Build history of the part. All positions in model axes, mm. A direction names the side the tool comes from. Round coordinates to 2 decimals unless told otherwise and drop trailing zeros. Order: outer loops, then holes, each group sorted by start corner. A loop starts at its lowest first (then second) coordinate and runs counter-clockwise, first axis right, second up. Notation, with made-up numbers: (-25, -26) -> (-9, -26) arc R8 ccw to (-9, -15) -> close; hole circle Ø4 at (73.5, 5). An arc over 180 degrees is marked (long way). Write item = value, one per line.
Autodesk Inventor part; units mm, degrees
ref_plane "Начальная плоскость" through (0, 0, -16.5685) normal (0, 0, 1) x (1, 0, 0)
ref_plane "Конечная плоскость" through (0, 0, 346.57) normal (0, 0, 1) x (1, 0, 0)
ref_plane "РабПлоскость4" through (21.07, -40, 346.57) normal (0, 0.7071, 0.7071) x (1, 0, 0)
ref_plane "Начальная плоскость" through (0, 0, -16.5685) normal (0, 0, 1) x (1, 0, 0)
ref_plane "Конечная плоскость" through (0, 0, 346.57) normal (0, 0, 1) x (1, 0, 0)
sketch "Эскиз" plane through (0, 0, 0) normal (0, 0, 1) x (1, 0, 0)
  line L0 (-1.43, 0) -> (-1.43, 40)
  line L1 (-1.43, 40) -> (43.57, 40)
  line L2 (43.57, 40) -> (43.57, 38.1774)
  line L3 (39.9881, 34.1993) -> (11.2338, 31.1771)
  line L4 (4.07, 23.221) -> (4.07, 0)
  line L5 (4.07, 0) -> (-1.43, 0) construction
  line L6 (23.82, 40) -> (23.82, 32.5) construction
  line L7 (43.57, 34.5758) -> (43.57, 32.5) construction
  line L8 (43.57, 32.5) -> (23.82, 32.5) construction
  line L9 (0, 15) -> (0, -27) construction
  line L10 (-5.539, 0) -> (16.0067, 0) construction
  line L11 (-1.43, 0) -> (-1.43, -40)
  line L12 (-1.43, -40) -> (43.57, -40)
  line L13 (43.57, -40) -> (43.57, -38.1774)
  line L14 (39.9881, -34.1993) -> (11.2338, -31.1771)
  line L15 (4.07, -23.221) -> (4.07, 0)
  arc A0 (11.2338, 31.1771) -> (4.07, 23.221) centre (12.07, 23.221) ccw
  arc A1 (4.07, -23.221) -> (11.2338, -31.1771) centre (12.07, -23.221) ccw
  arc A2 (39.9881, 34.1993) -> (43.57, 38.1774) centre (39.57, 38.1774) ccw
  arc A3 (43.57, -38.1774) -> (39.9881, -34.1993) centre (39.57, -38.1774) ccw
  line L16 (0, 56) -> (0, -56) construction
  line L17 (-15.5135, 0) -> (54.308, 0) construction
  point P0 (4.07, 30.4242)
  point P1 (43.57, -34.5758)
  point P2 (4.07, -30.4242)
  point P3 (23.82, -40)
  point P4 (23.82, -32.5)
  dimension "d0" = 5.5
  dimension "d1" = 40
  dimension "d2" = 45
  dimension "d3" = 7.5
  dimension "d4" = 19.75
  dimension "d5" = 2.0758
  dimension "d23" = 8
  dimension "d24" = 4
  dimension "d25" = 1.43
extrude "Тело" add sketch "Эскиз" along normal up to surface (363.1385 mm away) from surface at -16.5685
sketch "Sketch3" plane through (0, 0, 0) normal (0, 0, 1) x (1, 0, 0)
  line L0 (0, 0) -> (10, 0)
ref_plane "Work Plane3" through (0, 0, 0) normal (0, -1, 0) x (1, 0, 0)
sketch "Sketch4" plane through (0, 0, 0) normal (0, -1, 0) x (1, 0, 0)
  line L0 (-2, -16.5685) -> (12, -16.5685)
  line L1 (-2, 346.57) -> (12, 346.57)
  dimension "d29" = 363.1385
ref_plane "РабПлоскость4" through (21.07, -40, 346.57) normal (0, 0.7071, 0.7071) x (1, 0, 0)
split "Разделение1" plane through (21.07, -40, 346.57) removes the side toward (0, 0.7071, 0.7071)
ref_plane "РабПлоскость5" through (21.07, -40, -16.5685) normal (0, 0.3827, -0.9239) x (1, 0, 0)
split "Разделение2" plane through (21.07, -40, -16.5685) removes the side toward (0, 0.3827, -0.9239)
equation "\"d0\" = G_T"
equation "\"d1\" = 0.5 * G_H"
equation "\"d2\" = G_W"
equation "\"d3\" = G_T1"
equation "\"d4\" = G_C"
equation "\"d23\" = G_IR"
equation "\"d24\" = G_ER"
equation "\"d25\" = ex"
equation "\"d6\" = G_L"
equation "\"G_W\" = 45"
equation "\"G_T\" = 5.5"
equation "\"G_T1\" = 7.5"
equation "\"G_NG\" = 0.105104"
equation "\"G_ER\" = 4"
equation "\"G_IR\" = 8"
equation "\"G_C\" = 19.75"
equation "\"G_L\" = d29"
equation "\"ex\" = 1.43"
equation "\"G_OFFSET_START\" = 16.56854"
equation "\"d26\" = -G_OFFSET_START"
equation "\"d27\" = G_OFFSET_END + B_L"
equation "\"B_L\" = 306.57"
properties part number "ISO 657/11 - CH 80 x 8 - 363,14" material "Сталь, мягкая"
Q1. Cut at A-A, the plane z = 236.5. List the corners of the cut face in (x, y), and give its area (3 significant figures).
Check values:
outline = (-1.43, -40) -> (43.57, -40) -> (43.57, -38.18) arc R4 ccw to (39.99, -34.2) -> (11.23, -31.18) arc R8 cw to (4.07, -23.22) -> (4.07, 23.22) arc R8 cw to (11.23, 31.18) -> (39.99, 34.2) arc R4 ccw to (43.57, 38.18) -> (43.57, 40) -> (-1.43, 40) -> close
area = 1,050 mm²
Q2. Which spindle directions (+Z, -Z, +X, -X, +Y, -Y) get a long thin tool onto all of the face, cutting with end or side? Do faces 1 (the face through (25.81, -32.71, 160.82)), 2 (the face through (2.63, -0.19, 306.76)). Say none if no direction does.
Check values:
face_1 = +Z, -Z, +X
face_2 = +Z, +X, -X, +Y
Q3. Cut at D-D, the plane y = -14. List the corners of the cut face in (x, z).
Check values:
outline = (-1.43, -5.8) -> (4.07, -5.8) -> (4.07, 320.57) -> (-1.43, 320.57) -> close
Q4. Cut at C-C, the plane z = 296. List the corners of the cut face in (x, y), and give its area (3 significant figures).
Check values:
outline = (-1.43, -40) -> (43.57, -40) -> (43.57, -38.18) arc R4 ccw to (39.99, -34.2) -> (11.23, -31.18) arc R8 cw to (4.07, -23.22) -> (4.07, 10.57) -> (-1.43, 10.57) -> close
area = 582 mm²
Q5. Mould opens along Y. For faces 3 (the face through (4.07, 0, 158)), 4 (the face through (6.18, -28.635, 159.962)), 5 (the face through (21, 40, 140)), 6 (the face through (21, -40, 162)) say: released by +Y, released by -Y, zero draft, split by the parting line, or undercut.
Check values:
face_3 = undercut
face_4 = undercut
face_5 = released by +Y
face_6 = released by -Y
Q6. Cut at B-B, the plane x = 29.5. List the corners of the cut face in (y, z).
Check values:
outline = (-40, -16.57) -> (-33.1, -13.71) -> (-33.1, 339.67) -> (-40, 346.57) -> close; (33.1, 13.71) -> (40, 16.57) -> (40, 266.57) -> (33.1, 273.47) -> close
Q7. Probe probe 1 along X at (y, z) = (22.5, 104.5); probe 2 along Y at (x, z) = (22.5, 30.5); probe 3 along Y at (x, z) = (9, 266). List the from-to ranges inside material, lowest first.
Check values:
probe_1 = -1.43 to 4.07
probe_2 = -40 to -32.36, 32.36 to 40
probe_3 = -40 to -30.61, 30.61 to 40
Q8. Flat gauge pin, fed straight in: pin 1 (8 mm diameter, centred on y = 7.5, z = 65.5, fed in from +X). Where does the tip first touch, or does it go through?
Check values:
pin_1 = 4.07
